Work out the finished part from the listing and answer in its coordinate system (mm). Face numbers are marked on the shaded views. A direction names the side the tool comes from. Coordinates: 2 decimals unless noted, no trailing zeros. Loops run counter-clockwise (first coordinate to the right, second up) from the corner with the lowest first, then second, coordinate; pieces in that order, holes last. Notation, with made-up numbers: (17.5, 15.5) -> (23.5, 15.5) arc R28 ccw to (23.5, 47.5) -> close; hole circle Ø6 at (22, -25.5). An arc over 180 degrees is marked (long way). Answer as CSV lines item,"result".
```python
from build123d import *

# Parameters (mm, degrees)
Y_KSEKLIK_EKSTR_ZYON1_DEPTH = 3.5
IZIM2_R                     = 3.5
IZIM2_R_2                   = 0.5
Y_KSEKLIK_EKSTR_ZYON2_DEPTH = 0.5
IZIM3_R                     = 3.5
Y_KSEKLIK_EKSTR_ZYON3_DEPTH = 4.5
Y_KSEKLIK_EKSTR_ZYON4_DEPTH = 1
Y_KSEKLIK_EKSTR_ZYON5_DEPTH = 1
RADYUS1_R                   = 0.5


with BuildPart() as part:
    # Çizim1 → Yükseklik-Ekstrüzyon1 (new body)
    with BuildSketch(Plane.XY):
        with BuildLine():
            Line((0.5, 0), (11.5, 0))
            ThreePointArc((11.5, 0), (11.853553391, 0.146446609), (12, 0.5))
            Line((12, 0.5), (12, 11.5))
            ThreePointArc((12, 11.5), (11.853553391, 11.853553391), (11.5, 12))
            Line((11.5, 12), (0.5, 12))
            ThreePointArc((0.5, 12), (0.146446609, 11.853553391), (0, 11.5))
            Line((0, 11.5), (0, 0.5))
            ThreePointArc((0, 0.5), (0.146446609, 0.146446609), (0.5, 0))
        make_face()
    extrude(amount=Y_KSEKLIK_EKSTR_ZYON1_DEPTH)

    # Çizim2 → Yükseklik-Ekstrüzyon2 (add)
    with BuildSketch(Plane.XY.offset(3.5)):
        with Locations(Location((6, 6, 0), (0, 0, 180))):
            Circle(IZIM2_R)
        with Locations(Location((10, 10, 0), (0, 0, 180))):
            Circle(IZIM2_R_2)
        with Locations(Location((2, 10, 0), (0, 0, 180))):
            Circle(IZIM2_R_2)
        with Locations(Location((2, 2, 0), (0, 0, 180))):
            Circle(IZIM2_R_2)
        with Locations(Location((10, 2, 0), (0, 0, 180))):
            Circle(IZIM2_R_2)
    extrude(amount=Y_KSEKLIK_EKSTR_ZYON2_DEPTH)

    # Çizim3 → Yükseklik-Ekstrüzyon3 (add)
    with BuildSketch(Plane.XY.offset(4)):
        with Locations(Location((6, 6, 0), (0, 0, 180))):
            Circle(IZIM3_R)
    extrude(amount=Y_KSEKLIK_EKSTR_ZYON3_DEPTH)

    # Çizim4 → Yükseklik-Ekstrüzyon4 (add)
    with BuildSketch(Plane(origin=(0, 3, 0), x_dir=(-1, 0, 0), z_dir=(0, -1, 0))):
        with BuildLine():
            Line((0, -1), (0.25, -1))
            ThreePointArc((0.25, -1), (0.426776695, -0.926776695), (0.5, -0.75))
            Line((0.5, -0.75), (0.5, 3))
            Line((0.5, 3), (1, 3))
            Line((1, 3), (1, -1.25))
            ThreePointArc((1, -1.25), (0.926776695, -1.426776695), (0.75, -1.5))
            Line((0.75, -1.5), (0, -1.5))
            Line((0, -1.5), (0, -1))
        make_face()
        with BuildLine():
            Line((-12, -1.5), (-12, -1))
            Line((-12, -1), (-12.25, -1))
            ThreePointArc((-12.25, -1), (-12.426776695, -0.926776695), (-12.5, -0.75))
            Line((-12.5, -0.75), (-12.5, 3))
            Line((-12.5, 3), (-13, 3))
            Line((-13, 3), (-13, -1.25))
            ThreePointArc((-13, -1.25), (-12.926776695, -1.426776695), (-12.75, -1.5))
            Line((-12.75, -1.5), (-12, -1.5))
        make_face()
    extrude(amount=-Y_KSEKLIK_EKSTR_ZYON4_DEPTH)

    # Çizim6 → Yükseklik-Ekstrüzyon5 (add)
    with BuildSketch(Plane(origin=(0, 8.5, 0), x_dir=(1, 0, 0), z_dir=(0, 1, 0))):
        with BuildLine():
            Line((13, -1.25), (13, 3))
            Line((13, 3), (12.5, 3))
            Line((12.5, 3), (12.5, -0.75))
            ThreePointArc((12.5, -0.75), (12.426776695, -0.926776695), (12.25, -1))
            Line((12.25, -1), (12, -1))
            Line((12, -1), (12, -1.5))
            Line((12, -1.5), (12.75, -1.5))
            ThreePointArc((12.75, -1.5), (12.926776695, -1.426776695), (13, -1.25))
        make_face()
        with BuildLine():
            Line((0, -1.5), (0, -1))
            Line((0, -1), (-0.25, -1))
            ThreePointArc((-0.25, -1), (-0.426776695, -0.926776695), (-0.5, -0.75))
            Line((-0.5, -0.75), (-0.5, 3))
            Line((-0.5, 3), (-1, 3))
            Line((-1, 3), (-1, -1.25))
            ThreePointArc((-1, -1.25), (-0.926776695, -1.426776695), (-0.75, -1.5))
            Line((-0.75, -1.5), (0, -1.5))
        make_face()
    extrude(amount=Y_KSEKLIK_EKSTR_ZYON5_DEPTH)

    # Radyus1
    radyus1_edges = [part.edges().sort_by_distance(p)[0] for p in [
        (9.5, 6, 8.5),
    ]]
    fillet(radyus1_edges, radius=RADYUS1_R)


solid = part.part
```
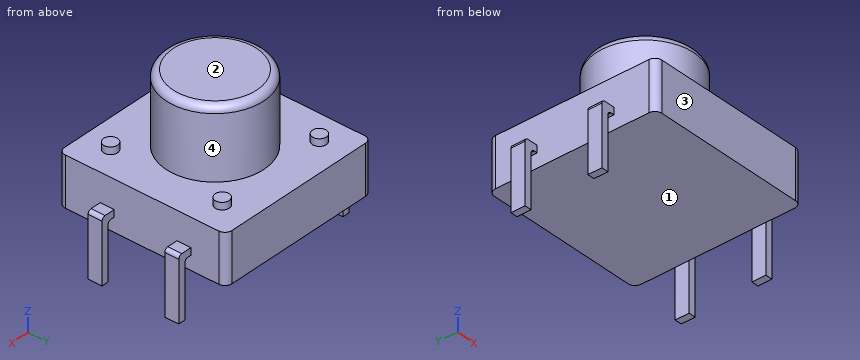
(1) A cutting plane is placed at D-D, the plane z = 1.75. Write down the section's boundary in (x, y).
Computed values:
outline,"(0, 0.5) arc R0.5 ccw to (0.5, 0) -> (11.5, 0) arc R0.5 ccw to (12, 0.5) -> (12, 11.5) arc R0.5 ccw to (11.5, 12) -> (0.5, 12) arc R0.5 ccw to (0, 11.5) -> close"
(2) Flat-ended cylindrical pins translate along their axes: pin 1 Ø4 at (x, y) = (10, 4.5) entering from -Z; pin 2 Ø0.6 at (x, y) = (12, 3.5) entering from +Z; pin 3 Ø0.5 at (x, y) = (2, 2) entering from +Z. Find the tip coordinate at first contact, or state that the pin passes through.
Computed values:
pin 1,"z = 0"
pin 2,"z = 3.5"
pin 3,"z = 4"
(3) A cutting plane is placed at A-A, the plane z = -0.75. Write down the section's boundary in (x, y).
Computed values:
outline,"(-1, 3) -> (-0.5, 3) -> (-0.5, 4) -> (-1, 4) -> close; (-1, 8.5) -> (-0.5, 8.5) -> (-0.5, 9.5) -> (-1, 9.5) -> close; (12.5, 3) -> (13, 3) -> (13, 4) -> (12.5, 4) -> close; (12.5, 8.5) -> (13, 8.5) -> (13, 9.5) -> (12.5, 9.5) -> close"
(4) Consider line 1 along Y through (x, z) = (12.75, -1); line 2 along Z through (x, y) = (11.75, 6.75); line 3 along X through (y, z) = (3.5, -1.5). Determine where each line is inside the solid, lowest interval first.
Computed values:
line 1,"3 to 4, 8.5 to 9.5"
line 2,"0 to 3.5"
line 3,"-1 to -0.5, 12.5 to 13"
(5) Which of the six approach directions +Z, -Z, +X, -X, +Y, -Y give full straight-line access (tool end or side, diameter ignored) to the marked faces 3 and 4?
Computed values:
face 3,"+Z, -Z, +X, -X, -Y"
face 4,"+Z"
(6) A cutting plane is placed at B-B, the plane y = 2. Write down the section's boundary in (x, z), and give its area (3 significant figures).
Computed values:
outline,"(0, 0) -> (12, 0) -> (12, 3.5) -> (10.5, 3.5) -> (10.5, 4) -> (9.5, 4) -> (9.5, 3.5) -> (2.5, 3.5) -> (2.5, 4) -> (1.5, 4) -> (1.5, 3.5) -> (0, 3.5) -> close"
area,"43.0 mm2"
(7) For a pull along X with two mould halves and no side action, classify the marked faces 1 and 2 as pulls with the +X half, pulls with the -X half, needs draft (parallel to the pull), parting line crosses it, or undercut.
Computed values:
face 1,"undercut"
face 2,"needs draft"
